from build123d import *

# Parameters (mm, degrees)
SKETCH2_R           = 1.6
SKETCH2_R_2         = 11.1
SKETCH2_R_3         = 3
SKETCH2_R_4         = 5
SKETCH2_R_5         = 4
BOSS_EXTRUDE1_DEPTH = 3


with BuildPart() as part:
    # Sketch2 → Boss-Extrude1 (new body)
    with BuildSketch(Plane.XY):
        with BuildLine():
            Line((614.435102185, 461.225170893), (623.90331335, 461.224719403))
            ThreePointArc((623.90331335, 461.224719403), (626.504195172, 461.509935711), (628.981434701, 462.352087069))
            Line((628.981434701, 462.352087069), (645.437814692, 472.74939936))
            Line((645.437814692, 472.74939936), (645.437805999, 475.842263452))
            ThreePointArc((645.437805999, 475.842263452), (645.827256367, 476.692258934), (646.675721819, 477.085031495))
            Line((646.675721819, 477.085031495), (651.053167865, 477.08497795))
            Line((651.053167865, 477.08497795), (658.053167865, 477.084892327))
            Line((658.053167865, 477.084892327), (661.05320456, 480.08485563))
            Line((661.05320456, 480.08485563), (661.053938478, 563.084855626))
            ThreePointArc((661.053938478, 563.084855626), (658.545785906, 568.910909563), (653.054048566, 572.084953481))
            Line((653.054048566, 572.084953481), (565.568648825, 572.225226264))
            ThreePointArc((565.568648825, 572.225226264), (557.08332923, 568.710610374), (553.568511969, 560.225374189))
            Line((553.568511969, 560.225374189), (553.568247664, 515.617572657))
            ThreePointArc((553.568247664, 515.617572657), (555.351154886, 509.323701089), (560.170211258, 504.900096998))
            Line((560.170211258, 504.900096998), (606.080895677, 487.576006806))
            Line((606.080895677, 487.576006806), (613.572105954, 487.575380074))
            ThreePointArc((613.572105954, 487.575380074), (613.822124483, 487.64230545), (614.005183481, 487.825274503))
            ThreePointArc((614.005183481, 487.825274503), (614.791773675, 487.928636269), (614.688030581, 487.142096277))
            ThreePointArc((614.688030581, 487.142096277), (614.504973528, 486.959127354), (614.437926006, 486.709143073))
            Line((614.437926006, 486.709143073), (614.43788575, 476.049724775))
            Line((614.43788575, 476.049724775), (624.220719005, 476.049608672))
            ThreePointArc((624.220719005, 476.049608672), (624.470734348, 476.116535454), (624.653790913, 476.299503103))
            ThreePointArc((624.653790913, 476.299503103), (625.440382085, 476.402865597), (625.336639048, 475.616324524))
            ThreePointArc((625.336639048, 475.616324524), (625.153582047, 475.433355654), (625.086534543, 475.183371443))
            Line((625.086534543, 475.183371443), (625.086160971, 473.615504488))
            ThreePointArc((625.086160971, 473.615504488), (625.15308783, 473.365488935), (625.336055679, 473.182432256))
            ThreePointArc((625.336055679, 473.182432256), (625.439417924, 472.395841553), (624.652877353, 472.499584586))
            ThreePointArc((624.652877353, 472.499584586), (624.46990843, 472.682641639), (624.219924149, 472.749689162))
            Line((624.219924149, 472.749689162), (614.437846894, 472.749804566))
            Line((614.437846894, 472.749804566), (614.435102185, 461.225170893))
        make_face()
        with Locations((635.087868744, 474.399923822)):
            Circle(SKETCH2_R, mode=Mode.SUBTRACT)
        with Locations((656.676324975, 488.487527015)):
            Circle(SKETCH2_R, mode=Mode.SUBTRACT)
        with Locations((625.676324975, 488.487527015)):
            Circle(SKETCH2_R, mode=Mode.SUBTRACT)
        with Locations((625.676324975, 534.094134141)):
            Circle(SKETCH2_R, mode=Mode.SUBTRACT)
        with Locations((641.176324975, 549.594134141)):
            Circle(SKETCH2_R_2, mode=Mode.SUBTRACT)
        with Locations((612.74313993, 513.399851045)):
            Circle(SKETCH2_R, mode=Mode.SUBTRACT)
        with Locations((656.676324975, 519.487527015)):
            Circle(SKETCH2_R, mode=Mode.SUBTRACT)
        with Locations((641.176324975, 503.987527015)):
            Circle(SKETCH2_R_2, mode=Mode.SUBTRACT)
        with Locations((625.676324975, 519.487527015)):
            Circle(SKETCH2_R, mode=Mode.SUBTRACT)
        with Locations((595.79313993, 557.52985104)):
            Circle(SKETCH2_R_3, mode=Mode.SUBTRACT)
        with Locations((656.676324975, 534.094134141)):
            Circle(SKETCH2_R, mode=Mode.SUBTRACT)
        with Locations((576.79313993, 519.52985104)):
            Circle(SKETCH2_R_4, mode=Mode.SUBTRACT)
        with Locations((579.79313993, 557.52985104)):
            Circle(SKETCH2_R_5, mode=Mode.SUBTRACT)
        with Locations((563.79313993, 557.52985104)):
            Circle(SKETCH2_R_3, mode=Mode.SUBTRACT)
        with Locations((625.676324975, 565.094134141)):
            Circle(SKETCH2_R, mode=Mode.SUBTRACT)
        with Locations((656.676324975, 565.094134141)):
            Circle(SKETCH2_R, mode=Mode.SUBTRACT)
        with BuildLine():
            Line((611.093697619, 549.224479725), (611.093697619, 540.09139539))
            ThreePointArc((611.093697619, 540.09139539), (611.02668037, 539.841343608), (610.843593883, 539.658322999))
            ThreePointArc((610.843593883, 539.658322999), (610.739850849, 538.871781922), (611.526442023, 538.975144428))
            ThreePointArc((611.526442023, 538.975144428), (611.709498586, 539.158112071), (611.959513926, 539.225038851))
            Line((611.959513926, 539.225038851), (613.527379805, 539.225038851))
            ThreePointArc((613.527379805, 539.225038851), (613.777380678, 539.158051129), (613.960393664, 538.975037363))
            ThreePointArc((613.960393664, 538.975037363), (614.746958334, 538.871481536), (614.643409294, 539.6580471))
            ThreePointArc((614.643409294, 539.6580471), (614.460398347, 539.841059611), (614.393411762, 540.091058378))
            Line((614.393411762, 540.091058378), (614.393411762, 549.224816737))
            ThreePointArc((614.393411762, 549.224816737), (614.460398347, 549.474815504), (614.643409294, 549.657828015))
            ThreePointArc((614.643409294, 549.657828015), (614.746958334, 550.444393579), (613.960393664, 550.340837752))
            ThreePointArc((613.960393664, 550.340837752), (613.777380678, 550.157823986), (613.527379805, 550.090836264))
            Line((613.527379805, 550.090836264), (611.959513926, 550.090836264))
            ThreePointArc((611.959513926, 550.090836264), (611.709498586, 550.157763044), (611.526442023, 550.340730687))
            ThreePointArc((611.526442023, 550.340730687), (610.739850849, 550.444093193), (610.843593883, 549.657552116))
            ThreePointArc((610.843593883, 549.657552116), (611.02668037, 549.474531507), (611.093697619, 549.224479725))
        make_face(mode=Mode.SUBTRACT)
    extrude(amount=BOSS_EXTRUDE1_DEPTH)


solid = part.part
Work out the finished part from the listing and answer in its coordinate system (mm). A direction names the side the tool comes from. Give positions to 0.01 mm unless a question says otherwise; leave off trailing zeros. Order: outer loops, then holes, each group sorted by start corner. A loop starts at its lowest first (then second) coordinate and runs counter-clockwise, first axis right, second up. Notation, with made-up numbers: (51, -32) - (103, -32) arc R22 ccw to (103, -21) - close; hole circle Ø4 at (-16, -27.75). An arc over 180 degrees is marked (long way). Answer as CSV lines item,"result". Start each with the question number.
Q1. Given pin 1 Ø0.9 at (x, z) = (656, 1) entering from -Y; pin 2 Ø0.5 at (y, z) = (474.5, 2) entering from -X; pin 3 Ø1.5 at (x, z) = (642, 1.5) entering from -Y; pin 4 Ø0.8 at (x, y) = (611.09, 539.23) entering from -Z, each flat-ended and moving along its own axis, determine where each tip first touches the part or whether it passes through.
Q2. For faces 1 (the face through (557.177, 568.803, 1.479)), 2 (the face through (614.393, 545, 1)), determine the directions among +Z, -Z, +X, -X, +Y, -Y from which every point of the face is accessible in a straight line to the end or side of a thin tool.
Q3. The part is cut by section A-A (y = 546). Write down the section's boundary in (x, z), then the cut area to 3 significant figures.
Q4. The part is cut by section C-C (x = 649). Write down the section's boundary in (y, z) (3 decimals).
Q5. The part is cut by section B-B (x = 574). Write down the section's boundary in (y, z).
Q6. The mould has two halves that part along X. Classify faces 3 (the face through (566.655, 558.431, 1.479)), 4 (the face through (555.303, 509.403, 1.479)): +X half, -X half, draft (parallel to the pull), parting line (faces both ways), or undercut.
Q7. Find the intervals of material crossed by L1, parallel to Y at x = 611.5, z = 0.9; L2, parallel to Y at x = 634, z = 1.55; L3, parallel to Y at x = 649, z = 0.65 (3 decimals), in increasing order. Write a range as [from, to].
Q8. The part is cut by section D-D (z = 1.2). Give the number of separate pieces and of enclosed holes in the cut face, then the cut area to 3 significant figures.
Check result:
1,pin 1,"stops at y = 477.08"
1,pin 2,"stops at x = 625.09"
1,pin 3,"stops at y = 470.1"
1,pin 4,"passes through"
2,face 1,"+Z, -Z, -X, +Y"
2,face 2,"+Z, -Z"
3,outline,"(553.57, 0) - (611.09, 0) - (611.09, 3) - (553.57, 3) - close; (614.39, 0) - (630.67, 0) - (630.67, 3) - (614.39, 3) - close; (651.68, 0) - (661.05, 0) - (661.05, 3) - (651.68, 3) - close"
3,area,"250 mm²"
4,outline,"(477.085, 0) - (496.114, 0) - (496.114, 3) - (477.085, 3) - close; (511.862, 0) - (541.72, 0) - (541.72, 3) - (511.862, 3) - close; (557.468, 0) - (572.091, 0) - (572.091, 3) - (557.468, 3) - close"
5,outline,"(499.68, 0) - (515.38, 0) - (515.38, 3) - (499.68, 3) - close; (523.68, 0) - (572.21, 0) - (572.21, 3) - (523.68, 3) - close"
6,face 3,"undercut"
6,face 4,"-X half"
7,L1,"y = [487.58, 512.39], [514.41, 538.93], [550.38, 572.15]"
7,L2,"y = [465.52, 473.23], [475.57, 495.52], [512.46, 541.13], [558.06, 572.12]"
7,L3,"y = [477.085, 496.114], [511.862, 541.72], [557.468, 572.091]"
8,separate pieces,"1"
8,enclosed holes,"17"
8,area,"8,260 mm²"
